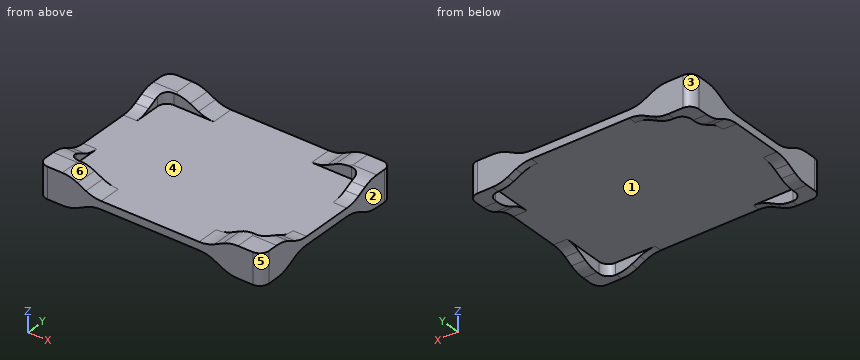
```python
from build123d import *

# Parameters (mm, degrees)
F2_DEPTH      = 8.5
F2_DEPTH_BACK = 5
F3_DEPTH      = 5
F5_START      = -3.5
F5_DEPTH      = 5
F7_DEPTH      = 98.001
F9_DEPTH      = 74.001
F10_T1_DEPTH  = 6.0466451645
F10_T3_DEPTH  = 6
F10_T5_DEPTH  = 3.25
F10_T7_DEPTH  = 3.5113155246
F10_T9_DEPTH  = 6
F10_T11_DEPTH = 9.75
F10_T13_DEPTH = 9.75
F10_T15_DEPTH = 23.7050983125
F10_T17_DEPTH = 23.751743477
F10_T19_DEPTH = 21.2164138371
F10_T21_DEPTH = 20.9550983125
F10_T23_DEPTH = 24.10822467
F10_T25_DEPTH = 24.10822467
F10_T27_DEPTH = 27.4550983125
F10_T29_DEPTH = 27.4550983125


# Not quite as in the source:
# - a fillet or chamfer that OpenCascade refuses, or shapes differently, is made with other operations: its cross-section is extruded or revolved along the edge and cut away or added


with BuildPart() as f2:
    # F1 (on Top) → F2 (new body, two sides)
    with BuildSketch(Plane.XY) as f2_sk:
        with BuildLine():
            ThreePointArc((-6, -5.75), (-4.8284271247, -8.5784271247), (-2, -9.75))
            Line((-2, -9.75), (88, -9.75))
            ThreePointArc((88, -9.75), (90.8284271247, -8.5784271247), (92, -5.75))
            Line((92, -5.75), (92, 60.25))
            ThreePointArc((92, 60.25), (90.8284271247, 63.0784271247), (88, 64.25))
            Line((88, 64.25), (-2, 64.25))
            ThreePointArc((-2, 64.25), (-4.8284271247, 63.0784271247), (-6, 60.25))
            Line((-6, 60.25), (-6, -5.75))
        make_face()
    extrude(amount=-F2_DEPTH)
    extrude(f2_sk.sketch, amount=F2_DEPTH_BACK)

    # F0 (on Top) → F3 (cut)
    with BuildSketch(Plane.XY):
        with BuildLine():
            ThreePointArc((0, 4), (1.1715728753, 1.1715728753), (4, 0))
            Line((4, 0), (82, 0))
            ThreePointArc((82, 0), (84.8284271247, 1.1715728753), (86, 4))
            Line((86, 4), (86, 50.5))
            ThreePointArc((86, 50.5), (84.8284271247, 53.3284271247), (82, 54.5))
            Line((82, 54.5), (4, 54.5))
            ThreePointArc((4, 54.5), (1.1715728753, 53.3284271247), (0, 50.5))
            Line((0, 50.5), (0, 4))
        make_face()
    extrude(amount=F3_DEPTH, mode=Mode.SUBTRACT)

    # F4 (on Top) → F5 (cut)
    with BuildSketch(Plane.XY.offset(F5_START)):
        with BuildLine():
            ThreePointArc((0, -2.5), (1.1715728753, -5.3284271247), (4, -6.5))
            Line((4, -6.5), (81.9533548355, -6.5))
            ThreePointArc((81.9533548355, -6.5), (84.7817819603, -5.3284271247), (85.9533548355, -2.5))
            Line((85.9533548355, -2.5), (85.9533548355, 56.7386844754))
            ThreePointArc((85.9533548355, 56.7386844754), (84.7817819603, 59.5671116002), (81.9533548355, 60.7386844754))
            Line((81.9533548355, 60.7386844754), (4, 60.7386844754))
            ThreePointArc((4, 60.7386844754), (1.1715728753, 59.5671116002), (0, 56.7386844754))
            Line((0, 56.7386844754), (0, -2.5))
        make_face()
    extrude(amount=-F5_DEPTH, mode=Mode.SUBTRACT)

    # F6 (on face) → F7 (cut, through all)
    with BuildSketch(Plane(origin=(-6, 0, 0), x_dir=(0, -1, 0), z_dir=(-1, 0, 0))):
        Polygon((-27.25, -8.5), (-2.25, -8.5), (-12.25, -3.5), (-27.25, -3.5), (-42.25, -3.5), (-52.25, -8.5), align=None)
        Polygon((-12.25, 0), (-2.25, 5), (-27.25, 5), (-52.25, 5), (-42.25, 0), (-27.25, 0), align=None)
    extrude(amount=-F7_DEPTH, mode=Mode.SUBTRACT)

    # F8 (on face) → F9 (cut, through all)
    with BuildSketch(Plane.XZ.offset(9.75)):
        Polygon((18, -3.5), (8, -8.5), (78, -8.5), (68, -3.5), (43, -3.5), align=None)
        Polygon((78, 5), (8, 5), (18, 0), (43, 0), (68, 0), align=None)
    extrude(amount=-F9_DEPTH, mode=Mode.SUBTRACT)

    # F10: fillet of radius 15 on 32 edges, made by hand

    # F10_s2 → F10_t1 (join)
    with BuildSketch(Plane.YZ.offset(85.9533548355)):
        with BuildLine():
            ThreePointArc((38.7089803375, -3.5), (42.1552741457, -3.901265158), (45.41718427, -5.083592135))
            Line((45.41718427, -5.083592135), (42.25, -3.5))
            Line((42.25, -3.5), (38.7089803375, -3.5))
        make_face()
        with BuildLine():
            ThreePointArc((15.7910196625, -3.5), (12.3447258543, -3.901265158), (9.08281573, -5.083592135))
            Line((9.08281573, -5.083592135), (12.25, -3.5))
            Line((12.25, -3.5), (15.7910196625, -3.5))
        make_face()
    extrude(amount=F10_T1_DEPTH)

    # F10_s4 → F10_t3 (join)
    with BuildSketch(Plane.YZ.offset(-6)):
        with BuildLine():
            ThreePointArc((38.7089803375, -3.5), (42.1552741457, -3.901265158), (45.41718427, -5.083592135))
            Line((45.41718427, -5.083592135), (42.25, -3.5))
            Line((42.25, -3.5), (38.7089803375, -3.5))
        make_face()
        with BuildLine():
            ThreePointArc((9.08281573, -5.083592135), (12.3447258543, -3.901265158), (15.7910196625, -3.5))
            Line((15.7910196625, -3.5), (12.25, -3.5))
            Line((12.25, -3.5), (9.08281573, -5.083592135))
        make_face()
        with BuildLine():
            ThreePointArc((15.7910196625, 0), (12.3447258543, 0.401265158), (9.08281573, 1.583592135))
            Line((9.08281573, 1.583592135), (12.25, 0))
            Line((12.25, 0), (15.7910196625, 0))
        make_face()
        with BuildLine():
            ThreePointArc((45.41718427, 1.583592135), (42.1552741457, 0.401265158), (38.7089803375, 0))
            Line((38.7089803375, 0), (42.25, 0))
            Line((42.25, 0), (45.41718427, 1.583592135))
        make_face()
    extrude(amount=F10_T3_DEPTH)

    # F10_s6 → F10_t5 (join)
    with BuildSketch(Plane.XZ.offset(6.5)):
        with BuildLine():
            ThreePointArc((64.4589803375, -3.5), (67.9052741457, -3.901265158), (71.16718427, -5.083592135))
            Line((71.16718427, -5.083592135), (68, -3.5))
            Line((68, -3.5), (64.4589803375, -3.5))
        make_face()
        with BuildLine():
            ThreePointArc((21.5410196625, -3.5), (18.0947258543, -3.901265158), (14.83281573, -5.083592135))
            Line((14.83281573, -5.083592135), (18, -3.5))
            Line((18, -3.5), (21.5410196625, -3.5))
        make_face()
    extrude(amount=F10_T5_DEPTH)

    # F10_s8 → F10_t7 (join)
    with BuildSketch(Plane.XZ.offset(-64.25)):
        with BuildLine():
            ThreePointArc((64.4589803375, -3.5), (67.9052741457, -3.901265158), (71.16718427, -5.083592135))
            Line((71.16718427, -5.083592135), (68, -3.5))
            Line((68, -3.5), (64.4589803375, -3.5))
        make_face()
        with BuildLine():
            ThreePointArc((21.5410196625, -3.5), (18.0947258543, -3.901265158), (14.83281573, -5.083592135))
            Line((14.83281573, -5.083592135), (18, -3.5))
            Line((18, -3.5), (21.5410196625, -3.5))
        make_face()
    extrude(amount=F10_T7_DEPTH)

    # F10_s10 → F10_t9 (join)
    with BuildSketch(Plane.YZ.offset(86)):
        with BuildLine():
            ThreePointArc((15.7910196625, 0), (12.3447258543, 0.401265158), (9.08281573, 1.583592135))
            Line((9.08281573, 1.583592135), (12.25, 0))
            Line((12.25, 0), (15.7910196625, 0))
        make_face()
        with BuildLine():
            ThreePointArc((38.7089803375, 0), (42.1552741457, 0.401265158), (45.41718427, 1.583592135))
            Line((45.41718427, 1.583592135), (42.25, 0))
            Line((42.25, 0), (38.7089803375, 0))
        make_face()
    extrude(amount=F10_T9_DEPTH)

    # F10_s12 → F10_t11 (join)
    with BuildSketch(Plane.XZ.offset(-64.25)):
        with BuildLine():
            ThreePointArc((64.4589803375, 0), (67.9052741457, 0.401265158), (71.16718427, 1.583592135))
            Line((71.16718427, 1.583592135), (68, 0))
            Line((68, 0), (64.4589803375, 0))
        make_face()
        with BuildLine():
            ThreePointArc((21.5410196625, 0), (18.0947258543, 0.401265158), (14.83281573, 1.583592135))
            Line((14.83281573, 1.583592135), (18, 0))
            Line((18, 0), (21.5410196625, 0))
        make_face()
    extrude(amount=F10_T11_DEPTH)

    # F10_s14 → F10_t13 (join)
    with BuildSketch(Plane.XZ):
        with BuildLine():
            ThreePointArc((64.4589803375, 0), (67.9052741457, 0.401265158), (71.16718427, 1.583592135))
            Line((71.16718427, 1.583592135), (68, 0))
            Line((68, 0), (64.4589803375, 0))
        make_face()
        with BuildLine():
            ThreePointArc((21.5410196625, 0), (18.0947258543, 0.401265158), (14.83281573, 1.583592135))
            Line((14.83281573, 1.583592135), (18, 0))
            Line((18, 0), (21.5410196625, 0))
        make_face()
    extrude(amount=F10_T13_DEPTH)

    # F10_s16 → F10_t15 (cut)
    with BuildSketch(Plane.YZ.offset(-14.8525491562)):
        with BuildLine():
            ThreePointArc((-1.2910196625, -8.5), (2.1552741457, -8.098734842), (5.41718427, -6.916407865))
            Line((5.41718427, -6.916407865), (2.25, -8.5))
            Line((2.25, -8.5), (-1.2910196625, -8.5))
        make_face()
        with BuildLine():
            ThreePointArc((49.08281573, -6.916407865), (52.3447258543, -8.098734842), (55.7910196625, -8.5))
            Line((55.7910196625, -8.5), (52.25, -8.5))
            Line((52.25, -8.5), (49.08281573, -6.916407865))
        make_face()
    extrude(amount=F10_T15_DEPTH, mode=Mode.SUBTRACT)

    # F10_s18 → F10_t17 (cut)
    with BuildSketch(Plane.YZ.offset(77.1008056793)):
        with BuildLine():
            ThreePointArc((5.41718427, -6.916407865), (2.1552741457, -8.098734842), (-1.2910196625, -8.5))
            Line((-1.2910196625, -8.5), (2.25, -8.5))
            Line((2.25, -8.5), (5.41718427, -6.916407865))
        make_face()
        with BuildLine():
            ThreePointArc((49.08281573, -6.916407865), (52.3447258543, -8.098734842), (55.7910196625, -8.5))
            Line((55.7910196625, -8.5), (52.25, -8.5))
            Line((52.25, -8.5), (49.08281573, -6.916407865))
        make_face()
    extrude(amount=F10_T17_DEPTH, mode=Mode.SUBTRACT)

    # F10_s20 → F10_t19 (cut)
    with BuildSketch(Plane.XZ.offset(-73.1025491562)):
        with BuildLine():
            ThreePointArc((74.83281573, -6.916407865), (78.0947258543, -8.098734842), (81.5410196625, -8.5))
            Line((81.5410196625, -8.5), (78, -8.5))
            Line((78, -8.5), (74.83281573, -6.916407865))
        make_face()
        with BuildLine():
            ThreePointArc((11.16718427, -6.916407865), (7.9052741457, -8.098734842), (4.4589803375, -8.5))
            Line((4.4589803375, -8.5), (8, -8.5))
            Line((8, -8.5), (11.16718427, -6.916407865))
        make_face()
    extrude(amount=F10_T19_DEPTH, mode=Mode.SUBTRACT)

    # F10_s22 → F10_t21 (cut)
    with BuildSketch(Plane.XZ.offset(-2.3525491562)):
        with BuildLine():
            ThreePointArc((74.83281573, -6.916407865), (78.0947258543, -8.098734842), (81.5410196625, -8.5))
            Line((81.5410196625, -8.5), (78, -8.5))
            Line((78, -8.5), (74.83281573, -6.916407865))
        make_face()
        with BuildLine():
            ThreePointArc((11.16718427, -6.916407865), (7.9052741457, -8.098734842), (4.4589803375, -8.5))
            Line((4.4589803375, -8.5), (8, -8.5))
            Line((8, -8.5), (11.16718427, -6.916407865))
        make_face()
    extrude(amount=F10_T21_DEPTH, mode=Mode.SUBTRACT)

    # F10_s24 → F10_t23 (cut)
    with BuildSketch(Plane.YZ.offset(-14.8525491562)):
        with BuildLine():
            ThreePointArc((5.41718427, 3.416407865), (2.1552741457, 4.598734842), (-1.2910196625, 5))
            Line((-1.2910196625, 5), (2.25, 5))
            Line((2.25, 5), (5.41718427, 3.416407865))
        make_face()
        with BuildLine():
            ThreePointArc((55.7910196625, 5), (52.3447258543, 4.598734842), (49.08281573, 3.416407865))
            Line((49.08281573, 3.416407865), (52.25, 5))
            Line((52.25, 5), (55.7910196625, 5))
        make_face()
    extrude(amount=F10_T23_DEPTH, mode=Mode.SUBTRACT)

    # F10_s26 → F10_t25 (cut)
    with BuildSketch(Plane.YZ.offset(76.7443244862)):
        with BuildLine():
            ThreePointArc((-1.2910196625, 5), (2.1552741457, 4.598734842), (5.41718427, 3.416407865))
            Line((5.41718427, 3.416407865), (2.25, 5))
            Line((2.25, 5), (-1.2910196625, 5))
        make_face()
        with BuildLine():
            ThreePointArc((55.7910196625, 5), (52.3447258543, 4.598734842), (49.08281573, 3.416407865))
            Line((49.08281573, 3.416407865), (52.25, 5))
            Line((52.25, 5), (55.7910196625, 5))
        make_face()
    extrude(amount=F10_T25_DEPTH, mode=Mode.SUBTRACT)

    # F10_s28 → F10_t27 (cut)
    with BuildSketch(Plane.XZ.offset(-73.1025491562)):
        with BuildLine():
            ThreePointArc((81.5410196625, 5), (78.0947258543, 4.598734842), (74.83281573, 3.416407865))
            Line((74.83281573, 3.416407865), (78, 5))
            Line((78, 5), (81.5410196625, 5))
        make_face()
        with BuildLine():
            ThreePointArc((4.4589803375, 5), (7.9052741457, 4.598734842), (11.16718427, 3.416407865))
            Line((11.16718427, 3.416407865), (8, 5))
            Line((8, 5), (4.4589803375, 5))
        make_face()
    extrude(amount=F10_T27_DEPTH, mode=Mode.SUBTRACT)

    # F10_s30 → F10_t29 (cut)
    with BuildSketch(Plane.XZ.offset(-8.8525491562)):
        with BuildLine():
            ThreePointArc((81.5410196625, 5), (78.0947258543, 4.598734842), (74.83281573, 3.416407865))
            Line((74.83281573, 3.416407865), (78, 5))
            Line((78, 5), (81.5410196625, 5))
        make_face()
        with BuildLine():
            ThreePointArc((11.16718427, 3.416407865), (7.9052741457, 4.598734842), (4.4589803375, 5))
            Line((4.4589803375, 5), (8, 5))
            Line((8, 5), (11.16718427, 3.416407865))
        make_face()
    extrude(amount=F10_T29_DEPTH, mode=Mode.SUBTRACT)


solid = f2.part
```
Model file for the job. Use its own axes, mm. Face numbers are marked on the shaded views. A direction names the side the tool comes from. Give positions to 0.01 mm unless a question says otherwise; leave off trailing zeros. Loops run counter-clockwise (first coordinate to the right, second up) from the corner with the lowest first, then second, coordinate; pieces in that order, holes last. Notation, with made-up numbers: (-5, -6.75) - (8, -6.75) arc R28 cw to (8, 16.25) - close; hole circle Ø1 at (51, -17). An arc over 180 degrees is marked (long way). One line per item, written item: value. Start each with the question number.
1. Which spindle directions (+Z, -Z, +X, -X, +Y, -Y) get a long thin tool onto all of the face, cutting with end or side? Do the marked faces 4, 5 and 6. Say none if no direction does.
2. Slice it at A-A (x = 68.5). List the corners of the cut face in (y, z).
3. Pull direction X, two halves, no side cores. Call the marked faces 1, 2 and 3: pulls with the +X half, pulls with the -X half, needs draft (parallel to the pull), parting line crosses it, or undercut.
4. Pin check, flat tips, straight feed: pin 1 (5 mm diameter, centred on x = 22.5, y = 30, fed in from +Z); pin 2 (22 mm diameter, centred on x = 37.5, y = 16.5, fed in from -Z); pin 3 (2 mm diameter, centred on x = 19, z = 2, fed in from +Y) (3 decimals). Stop position of each tip, or through.
5. Probe L1, parallel to Y at x = 78, z = 2.5; L2, parallel to Z at x = 7.5, y = 27.5. List the from-to ranges inside material, lowest first. Write a range as from..to.
6. Slice it at D-D (y = 29). List the corners of the cut face in (x, z), plus the area to 3 significant figures.
7. Slice it at B-B (y = 52). List the corners of the cut face in (x, z), plus the area to 3 significant figures.
8. Slice it at C-C (x = 49.5). List the corners of the cut face in (y, z).
Solution:
1. face 4: +Z
1. face 5: +Z, -Z, +X, -Y
1. face 6: +Z, +Y, -Y
2. outline: (-9.75, -4.05) - (-6.5, -4.05) - (-6.5, -3.5) - (60.74, -3.5) - (60.74, -4.05) - (64.25, -4.05) - (64.25, 0.55) - (54.5, 0.55) - (54.5, 0) - (0, 0) - (0, 0.55) - (-9.75, 0.55) - close
3. face 1: undercut
3. face 2: pulls with the +X half
3. face 3: pulls with the -X half
4. pin 1: stops at z = 0
4. pin 2: stops at z = -3.5
4. pin 3: passes through
5. L1: y = -9.75..0, 54.5..64.25
5. L2: z = -3.5..0
6. outline: (-6, -3.5) - (92, -3.5) - (92, 0) - (-6, 0) - close
6. area: 343 mm^2
7. outline: (-6, -8.01) - (0, -8.01) - (0, -3.5) - (85.95, -3.5) - (85.95, -8.01) - (92, -8.01) - (92, 4.51) - (85.71, 4.51) - (85.71, 0) - (0.29, 0) - (0.29, 4.51) - (-6, 4.51) - close
7. area: 454 mm^2
8. outline: (-9.75, -3.5) - (64.25, -3.5) - (64.25, 0) - (-9.75, 0) - close
